For this review, take the finished solid that the model builds, in its own axes (mm). A direction names the side the tool comes from. Give positions to 0.01 mm unless a question says otherwise; leave off trailing zeros. Order: outer loops, then holes, each group sorted by start corner. A loop starts at its lowest first (then second) coordinate and runs counter-clockwise, first axis right, second up. Notation, with made-up numbers: (10.25, -30) - (42.25, -30) arc R28 ccw to (42.25, -3) - close; hole circle Ø2 at (71, 17). An arc over 180 degrees is marked (long way). Use a Markdown table: item, result. Add a question column.
1) Clearance check with flat-ended pins moving along their axes: P1, Ø2, axis at x = 20, z = 3, coming from the -Y side; P2, Ø1.6, axis at x = 1, z = 1.5, coming from the -Y side; P3, Ø2, axis at y = 5.5, z = 2.5, coming from the -X side; P4, Ø2, axis at x = 11, y = -24.5, coming from the -Z side. State where each tip first meets the part, or that it passes through.
2) Machinability: for faces 5 (the face through (23, -57, 2)), 6 (the face through (5, 5, 2)), 7 (the face through (24, -35, 2)), which of the approach directions +Z, -Z, +X, -X, +Y, -Y give a long, thin tool a straight path to every point of the face, cutting with its end or side? Answer none if there is none.
3) We need section B-B on x = 21. Write out the cut boundary in (y, z), then the cut area to 3 significant figures.
4) We need section D-D on z = 3.3. Give the number of separate pieces and of enclosed holes in the cut face, then the cut area to 3 significant figures.
5) Wall thickness on L1, parallel to X at y = -28.5, z = 0.9; L2, parallel to Y at x = 21, z = 2.1; L3, parallel to Y at x = 0, z = 1.85: over which ranges is each line inside the solid? List them lowest first.
6) We need section C-C on y = 0. Write out the cut boundary in (x, z), then the cut area to 3 significant figures.
7) Mouldability with a two-part tool opening along Y and no side actions: class faces 1 (the face through (22, -47, 2)), 2 (the face through (22, -23, 2)), 3 (the face through (1, 3, 2)), 4 (the face through (5.57, -16.9, 1.97)) as released by +Y, released by -Y, zero draft, split by the parting line, or undercut.
8) We need section A-A on y = -26. Write out the cut boundary in (x, z).
```python
from build123d import *

# Parameters (mm, degrees)
SKETCH_1_W          = 15
SKETCH_1_H          = 6
SKETCH_1_W_2        = 25
SKETCH_1_R          = 1.5
SKETCH_1_W_3        = 4
SKETCH_1_H_2        = 10
EXTRUDE_1_DEPTH     = 4
CUT_EXTRUDE_1_DEPTH = 4
CHAMFER_1_SIZE      = 1.8
SKETCH_3_W          = 4
SKETCH_3_H          = 44
EXTRUDE_2_DEPTH     = 4
CUT_EXTRUDE_2_DEPTH = 4
FILLET_1_R          = 0.5
SKETCH_12_W         = 3
SKETCH_12_H         = 18.4
CUT_EXTRUDE_6_DEPTH = 10
CUT_EXTRUDE_7_DEPTH = 10
FILLET_2_R          = 5
FILLET_3_R          = 2


with BuildPart() as part:
    # 草图1 → 凸台-拉伸1 (new body)
    # profile 1 of 5: a face of its own
    with BuildSketch(Plane.XY):
        with Locations((12.5, 6)):
            Rectangle(SKETCH_1_W, SKETCH_1_H)
    # profile 2 of 5: a face of its own
    with BuildSketch(Plane.XY):
        with Locations((7.5, 0)):
            Rectangle(SKETCH_1_W_2, SKETCH_1_H)
        Circle(SKETCH_1_R, mode=Mode.SUBTRACT)
        with Locations((10, 0)):
            Circle(SKETCH_1_R, mode=Mode.SUBTRACT)
    # profile 3 of 5: a face of its own
    with BuildSketch(Plane.XY):
        Polygon((10, -65), (20, -65), (20, -3), (-5, -3), align=None)
    # profile 4 of 5: a face of its own
    with BuildSketch(Plane.XY):
        with Locations((22, -18)):
            Rectangle(SKETCH_1_W_3, SKETCH_1_H_2)
    # profile 5 of 5: a face of its own
    with BuildSketch(Plane.XY):
        with Locations((22, -52)):
            Rectangle(SKETCH_1_W_3, SKETCH_1_H_2)
    extrude(amount=EXTRUDE_1_DEPTH)

    # 草图2 → 切除-拉伸1 (cut)
    with BuildSketch(Plane.XY.offset(4)):
        with BuildLine():
            Line((20, -13), (20, -12))
            ThreePointArc((20, -12), (19.5, -12.5), (20, -13))
        make_face()
        with BuildLine():
            Line((20, -24), (20, -23))
            ThreePointArc((20, -23), (19.5, -23.5), (20, -24))
        make_face()
        with BuildLine():
            Line((20, -47), (20, -46))
            ThreePointArc((20, -46), (19.5, -46.5), (20, -47))
        make_face()
        with BuildLine():
            Line((20, -58), (20, -57))
            ThreePointArc((20, -57), (19.5, -57.5), (20, -58))
        make_face()
        with BuildLine():
            ThreePointArc((3.5, 3), (4.25, 2.25), (5, 3))
            Line((5, 3), (3.5, 3))
        make_face()
    extrude(amount=-CUT_EXTRUDE_1_DEPTH, mode=Mode.SUBTRACT)

    # 倒角1
    chamfer_1_edges = [part.edges().sort_by_distance(p)[0] for p in [
        (8.5, 0, 4),
    ]]
    chamfer(chamfer_1_edges, length=CHAMFER_1_SIZE)

    # 草图3 → 凸台-拉伸2 (add)
    with BuildSketch(Plane.XY.offset(4)):
        with Locations((26, -35)):
            Rectangle(SKETCH_3_W, SKETCH_3_H)
    extrude(amount=-EXTRUDE_2_DEPTH)

    # 草图4 → 切除-拉伸2 (cut)
    with BuildSketch(Plane.XY.offset(4)):
        with BuildLine():
            Line((24, -23), (24, -24))
            ThreePointArc((24, -24), (24.5, -23.5), (24, -23))
        make_face()
        with BuildLine():
            Line((24, -46), (24, -47))
            ThreePointArc((24, -47), (24.5, -46.5), (24, -46))
        make_face()
    extrude(amount=-CUT_EXTRUDE_2_DEPTH, mode=Mode.SUBTRACT)

    # 圆角1
    fillet_1_edges = [part.edges().sort_by_distance(p)[0] for p in [
        (24, -24, 2),
        (24, -46, 2),
        (20, -24, 2),
        (20, -46, 2),
        (20, -58, 2),
        (3.5, 3, 2),
        (20, -12, 2),
    ]]
    fillet(fillet_1_edges, radius=FILLET_1_R)

    # 草图12 → 切除-拉伸6 (cut)
    with BuildSketch(Plane.XY.offset(4)):
        with Locations((-3.5, -6.2)):
            Rectangle(SKETCH_12_W, SKETCH_12_H)
    extrude(amount=-CUT_EXTRUDE_6_DEPTH, mode=Mode.SUBTRACT)

    # 草图13 → 切除-拉伸7 (cut)
    with BuildSketch(Plane.XY.offset(4)):
        Polygon((7, -52.6), (-2, -15.4), (7, -15.4), align=None)
    extrude(amount=-CUT_EXTRUDE_7_DEPTH, mode=Mode.SUBTRACT)

    # 圆角2
    fillet_2_edges = [part.edges().sort_by_distance(p)[0] for p in [
        (7, -15.4, 2),
    ]]
    fillet(fillet_2_edges, radius=FILLET_2_R)

    # 圆角3
    fillet_3_edges = [part.edges().sort_by_distance(p)[0] for p in [
        (28, -13, 2),
        (28, -57, 2),
        (-2, -15.4, 2),
        (7, -52.6, 2),
        (5, 9, 2),
        (20, 9, 2),
        (20, -65, 2),
        (10, -65, 2),
    ]]
    fillet(fillet_3_edges, radius=FILLET_3_R)


solid = part.part
```
Checked values:
| question | item | result |
|---|---|---|
| 1 | P1 | y = -64.73 |
| 1 | P2 | y = -15.4 |
| 1 | P3 | x = 5 |
| 1 | P4 | z = 0 |
| 2 | face 5 | +Z, -Z, +X, -Y |
| 2 | face 6 | +Z, -Z, -X, +Y |
| 2 | face 7 | +Z, -Z |
| 3 | outline | (-57, 0) - (-47, 0) - (-47, 4) - (-57, 4) - close; (-23, 0) - (-13, 0) - (-13, 4) - (-23, 4) - close |
| 3 | area | 80.0 mm² |
| 4 | separate pieces | 1 |
| 4 | enclosed holes | 3 |
| 4 | area | 1,350 mm² |
| 5 | L1 | 7 to 20, 24 to 28 |
| 5 | L2 | -57 to -47, -23 to -13 |
| 5 | L3 | -15.4 to -1.5, 1.5 to 3 |
| 6 | outline | (-2, 0) - (-1.5, 0) - (-1.5, 4) - (-2, 4) - close; (1.5, 0) - (8.5, 0) - (8.5, 2.2) - (6.7, 4) - (1.5, 4) - close; (11.5, 0) - (20, 0) - (20, 4) - (13.3, 4) - (11.5, 2.2) - close |
| 6 | area | 60.8 mm² |
| 7 | face 1 | undercut |
| 7 | face 2 | undercut |
| 7 | face 3 | released by +Y |
| 7 | face 4 | released by -Y |
| 8 | outline | (7, 0) - (20, 0) - (20, 4) - (7, 4) - close; (24, 0) - (28, 0) - (28, 4) - (24, 4) - close |
